The model under review builds one solid part; all positions refer to its coordinate system, in mm. Face numbers are marked on the shaded views. A direction names the side the tool comes from. Coordinates: 2 decimals unless noted, no trailing zeros. Write each loop counter-clockwise with the first axis right and the second up, starting at its lowest first coordinate (ties: lowest second). Pieces come first, ordered by that corner, then holes. Notation, with made-up numbers: (9, 61) - (30, 61) arc R6 ccw to (30, 71) - close; hole circle Ø10 at (9, 41.5). An arc over 180 degrees is marked (long way). Put each result on its own line as item: value.
from build123d import *

# Parameters (mm, degrees)
BOSS_EXTRUDE3_DEPTH = 14
SKETCH4_R           = 0.575
BOSS_EXTRUDE4_DEPTH = 5
SKETCH5_R           = 2
BOSS_EXTRUDE5_DEPTH = 1


with BuildPart() as part:
    # Sketch1 → Boss-Extrude3 (new body)
    with BuildSketch(Plane.XY):
        Polygon((0, 0), (32, 0), (32, 21), (0, 21), (0, 14.5), (4.5, 14.5), (4.5, 16.5), (27.5, 16.5), (27.5, 4.5), (4.5, 4.5), (4.5, 6.5), (0, 6.5), align=None)
    extrude(amount=BOSS_EXTRUDE3_DEPTH)

    # Sketch4 → Boss-Extrude4 (add)
    with BuildSketch(Plane.XY.offset(14)):
        with Locations((29.7, 10.5)):
            Circle(SKETCH4_R)
    extrude(amount=BOSS_EXTRUDE4_DEPTH)

    # Sketch5 → Boss-Extrude5 (add)
    with BuildSketch(Plane.XY.offset(19)):
        with Locations((29.7, 10.5)):
            Circle(SKETCH5_R)
    extrude(amount=BOSS_EXTRUDE5_DEPTH)


solid = part.part
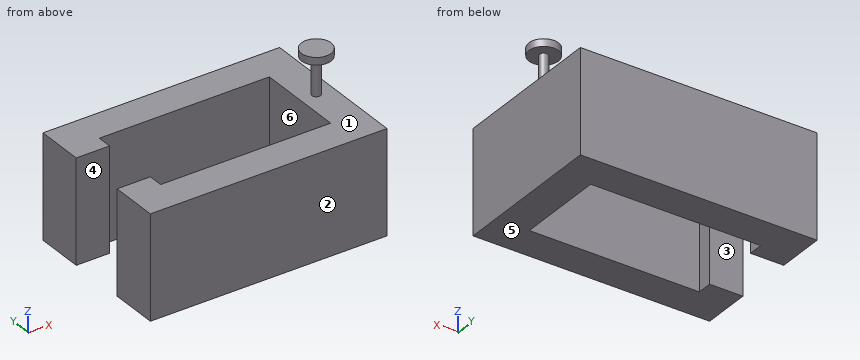
1. To check wall thickness, follow probe 1 along X at (y, z) = (16.25, 13); probe 2 along Y at (x, z) = (17, 12); probe 3 along X at (y, z) = (10.5, 4.5). State the ranges of each line that lie inside material, in increasing order.
Determined:
probe 1: x = 0 to 4.5, 27.5 to 32
probe 2: y = 0 to 4.5, 16.5 to 21
probe 3: x = 27.5 to 32
2. Machinability: for the marked faces 4, 5 and 6, which of the approach directions +Z, -Z, +X, -X, +Y, -Y give a long, thin tool a straight path to every point of the face, cutting with its end or side? Answer none if there is none.
Determined:
face 4: +Z, -Z, -X
face 5: -Z, +X, -X, +Y, -Y
face 6: +Z, -Z
3. For pin 1 Ø1.5 at (x, y) = (11.5, 5.5) entering from +Z; pin 2 Ø1.5 at (y, z) = (7.5, 7) entering from -X; pin 3 Ø2 at (x, y) = (28.5, 6) entering from +Z, all flat-tipped, find the tip position at first contact; note any pin that passes through.
Determined:
pin 1: passes through
pin 2: stops at x = 27.5
pin 3: stops at z = 14
4. Consider section A-A on y = 15.25. State the section outline as (x, z) points.
Determined:
outline: (0, 0) - (4.5, 0) - (4.5, 14) - (0, 14) - close; (27.5, 0) - (32, 0) - (32, 14) - (27.5, 14) - close
5. Consider section C-C on z = 7.25. State the section outline as (x, y) points, plus the area to 3 significant figures.
Determined:
outline: (0, 0) - (32, 0) - (32, 21) - (0, 21) - (0, 14.5) - (4.5, 14.5) - (4.5, 16.5) - (27.5, 16.5) - (27.5, 4.5) - (4.5, 4.5) - (4.5, 6.5) - (0, 6.5) - close
area: 360 mm^2
6. The part is to be moulded in two halves that separate along Y. For the marked faces 1, 2 and 3, say which applies: +Y half, -Y half, draft (parallel to the pull), parting line (faces both ways), or undercut.
Determined:
face 1: draft
face 2: -Y half
face 3: undercut
7. Consider section B-B on x = 21. State the section outline as (y, z) points, plus the area to 3 significant figures.
Determined:
outline: (0, 0) - (4.5, 0) - (4.5, 14) - (0, 14) - close; (16.5, 0) - (21, 0) - (21, 14) - (16.5, 14) - close
area: 126 mm^2
8. Consider section D-D on y = 10.5. State the section outline as (x, z) points (3 decimals), plus the area to 4 significant figures.
Determined:
outline: (27.5, 0) - (32, 0) - (32, 14) - (30.275, 14) - (30.275, 19) - (31.7, 19) - (31.7, 20) - (27.7, 20) - (27.7, 19) - (29.125, 19) - (29.125, 14) - (27.5, 14) - close
area: 72.75 mm^2
